Design review of the part shown in the three views and the two pictorial views. Dimensions are in mm from the part's minimum x, y and z. A direction names the side the tool comes from. Round coordinates to 2 decimals unless told otherwise and drop trailing zeros. Order: outer loops, then holes, each group sorted by start corner. A loop starts at its lowest first (then second) coordinate and runs counter-clockwise, first axis right, second up. Notation, with made-up numbers: (73.5, 55.25) - (107.5, 55.25) arc R11 cw to (107.5, 75.25) - close; hole circle Ø7 at (-10.5, 10). An arc over 180 degrees is marked (long way). One line per question, with ' | ' between items. Start each with the question number.
Item 1: Add section D-D on y = 15. State how many separate pieces and enclosed holes the cut face has, and give its area (3 significant figures).
Item 2: Draft analysis for pull direction Z (two halves, no side actions). For the marked faces 1, 2, 3 and 4, state which applies: +Z half, -Z half, draft (parallel to the pull), parting line (faces both ways), or undercut.
Item 3: For L1, parallel to Z at x = 26, y = 25; L2, parallel to Z at x = 3, y = 15 (3 decimals); L3, parallel to X at y = 14.5, z = 2, list the stretches that pass through material, from the lowest coordinate up. Write a range as [from, to].
Item 4: Add section A-A on z = 3. State the section outline as (x, y) points, and give its area (3 significant figures).
Item 5: Insertion check: pin 1 Ø3.5 at (x, y) = (16.5, 14) entering from -Z; pin 2 Ø9 at (x, z) = (15.5, 7.5) entering from -Y; pin 3 Ø4 at (y, z) = (6, 7) entering from -X; pin 4 Ø5 at (y, z) = (10, 19.5) entering from +X. Each pin has a flat end and moves straight along its axis. Give the tip position at first contact, or say it passes through.
Item 6: Add section C-C on z = 10. State the section outline as (x, y) points (3 decimals), and give its area (3 significant figures).
Item 7: Tool access review of the marked faces 5 and 6: name each direction out of +Z, -Z, +X, -X, +Y, -Y from which nothing blocks a thin tool from reaching the whole face with its end or side.
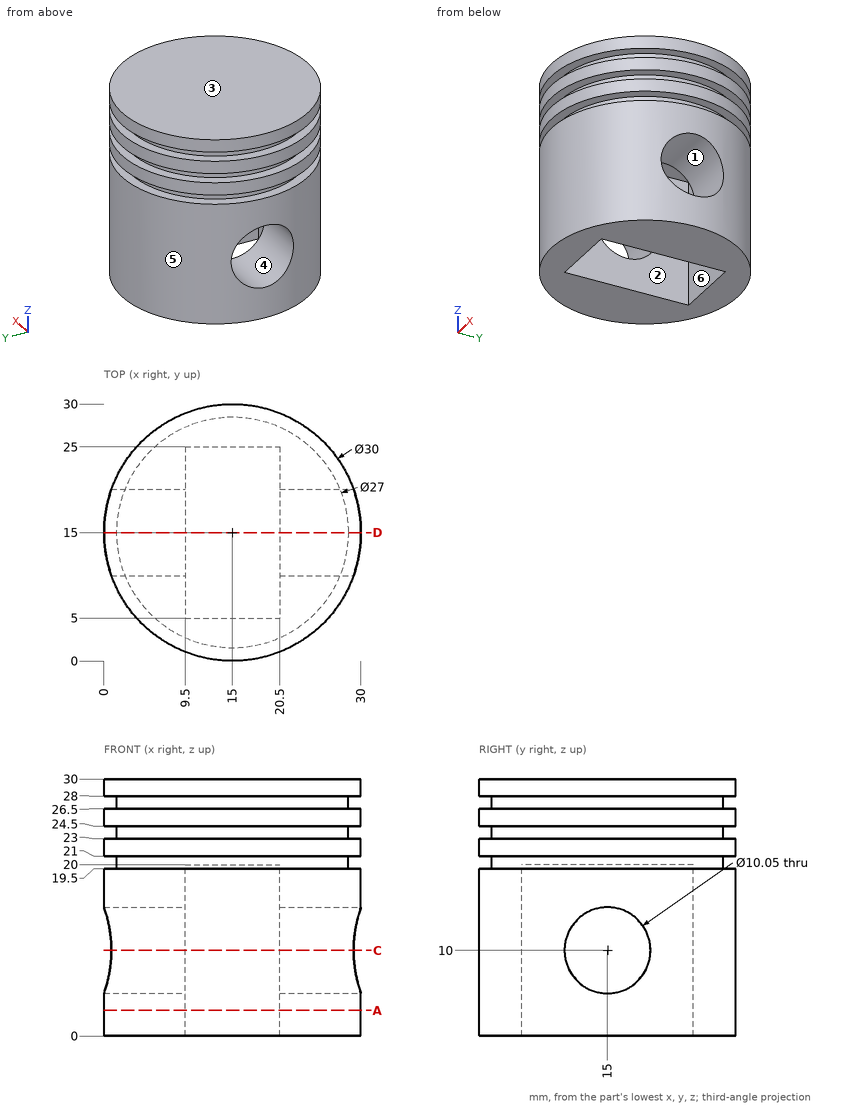
Determined:
1) separate pieces: 3 | enclosed holes: 0 | area: 476 mm2
2) face 1: undercut | face 2: draft | face 3: +Z half | face 4: undercut
3) L1: [0, 19.5], [21, 23], [24.5, 26.5], [28, 30] | L2: [0, 4.975], [15.025, 30] | L3: [0.01, 9.5], [20.5, 29.99]
4) outline: circle Ø30 at (15, 15); hole (9.5, 5) - (20.5, 5) - (20.5, 25) - (9.5, 25) - close | area: 487 mm2
5) pin 1: z = 20 | pin 2: y = 0 | pin 3: x = 1.73 | pin 4: x = 29.79
6) outline: (0.867, 9.975) arc R15 ccw to (29.133, 9.975) - (20.5, 9.975) - (20.5, 5) - (9.5, 5) - (9.5, 9.975) - close; (0.867, 20.025) - (9.5, 20.025) - (9.5, 25) - (20.5, 25) - (20.5, 20.025) - (29.133, 20.025) arc R15 ccw to start | area: 302 mm2
7) face 5: +Z, -Z | face 6: -Z
